Check sheet for the modelled part. Datum: model origin and axes. Units: mm. Face numbers are marked on the shaded views. A direction names the side the tool comes from. Coordinates: 2 decimals unless noted, no trailing zeros. Loops run counter-clockwise (first coordinate to the right, second up) from the corner with the lowest first, then second, coordinate; pieces in that order, holes last. Notation, with made-up numbers: (-35, 59) -> (-4, 59) arc R9 ccw to (-4, 74) -> close; hole circle Ø3 at (37.5, 33). An arc over 180 degrees is marked (long way). Use one line per item in the form item = value.
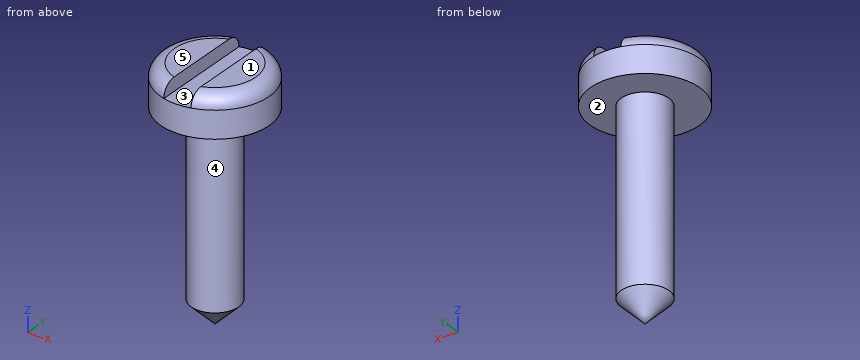
from build123d import *

# Parameters (mm, degrees)
SKICA1_R                 = 1.75
VYSUNOUT1_DEPTH          = 15
SKICA3_R                 = 4
VYSUNOUT2_DEPTH          = 3
ZAOBLIT1_R               = 1
ZKOSIT1_SIZE             = 1.75
SKICA8_W                 = 2
SKICA8_H                 = 8
ODEBRAT_VYSUNUT_M2_DEPTH = 1


with BuildPart() as part:
    # Skica1 → Vysunout1 (new body)
    with BuildSketch(Plane.XY):
        Circle(SKICA1_R)
    extrude(amount=VYSUNOUT1_DEPTH)

    # Skica3 → Vysunout2 (add)
    with BuildSketch(Plane.XY.offset(15)):
        Circle(SKICA3_R)
    extrude(amount=VYSUNOUT2_DEPTH)

    # Zaoblit1
    zaoblit1_edges = [part.edges().sort_by_distance(p)[0] for p in [
        (-4, 0, 18),
    ]]
    fillet(zaoblit1_edges, radius=ZAOBLIT1_R)

    # Zkosit1
    zkosit1_edges = [part.edges().sort_by_distance(p)[0] for p in [
        (-1.75, 0, 0),
    ]]
    chamfer(zkosit1_edges, length=ZKOSIT1_SIZE)

    # Skica8 → Odebrat vysunutím2 (cut)
    with BuildSketch(Plane.XY.offset(18)):
        Rectangle(SKICA8_W, SKICA8_H)
    extrude(amount=-ODEBRAT_VYSUNUT_M2_DEPTH, mode=Mode.SUBTRACT)


solid = part.part
(1) Tool access check on the marked faces 1 and 2. Record the directions out of +Z, -Z, +X, -X, +Y, -Y that give a thin tool (end or side, any length) a straight path to the whole face; none if there is none.
Established:
face_1 = +Z, +X, -X, +Y, -Y
face_2 = -Z
(2) Section check A-A, the plane z = 14. Record the boundary of the cut face in (x, y).
Established:
outline = circle Ø3.5 at (0, 0)
(3) Go/stop test with flat-tipped pins: P1, Ø1, axis at x = -1, z = 10.5, coming from the +Y side; P2, Ø2, axis at x = 2.5, z = 4, coming from the +Y side; P3, Ø3, axis at x = 2.5, y = 0, coming from the -Z side. Record where each tip stops, or that it passes through.
Established:
P1 = 1.68
P2 = 0.9
P3 = 1
(4) Scan lines: line 1 along Y through (x, z) = (0, 3); line 2 along Z through (x, y) = (-0.75, 1.75); line 3 along Z through (x, y) = (1.75, -1). Record each from-to range of solid material in increasing order.
Established:
line_1 = -1.75 to 1.75
line_2 = 15 to 17
line_3 = 15 to 18
(5) Mould release check, pull along X, two halves, no side actions. Record for the marked faces 3, 4 and 5: +X half, -X half, draft (parallel to the pull), parting line (faces both ways), or undercut.
Established:
face_3 = undercut
face_4 = parting line
face_5 = draft
